```python
from build123d import *

# Parameters (mm, degrees)
SKETCH1_R           = 16
SKETCH1_R_2         = 5
BOSS_EXTRUDE3_DEPTH = 70
CUT_EXTRUDE2_DEPTH  = 16
CUT_EXTRUDE3_DEPTH  = 16
SKETCH7_W           = 34
SKETCH7_H           = 251.612307305
CUT_EXTRUDE4_DEPTH  = 87.5
CUT_EXTRUDE5_DEPTH  = 34
BOSS_EXTRUDE4_START = -38
BOSS_EXTRUDE4_DEPTH = 38
CUT_EXTRUDE6_DEPTH  = 135


with BuildPart() as part:
    # Sketch1 → Boss-Extrude3 (new body)
    with BuildSketch(Plane.XY):
        with BuildLine():
            Line((-18.492879119, 133.036316601), (-18.498498023, 133.025878551))
            ThreePointArc((-18.498498023, 133.025878551), (-22.931133945, 136.748933151), (-27.911859958, 139.698808598))
            Line((-27.911859958, 139.698808598), (-28.859852333, 137.937754807))
            ThreePointArc((-28.859852333, 137.937754807), (-24.623995913, 135.183968868), (-20.885371833, 131.785659496))
            ThreePointArc((-20.885371833, 131.785659496), (-18.192980361, 129.380347747), (-15.794912153, 126.681502565))
            Line((-15.794912153, 126.681502565), (-27.917185271, 110.194914382))
            Line((-27.917185271, 110.194914382), (-24.189891295, 89.250297825))
            ThreePointArc((-24.189891295, 89.250297825), (-23.276240724, 85.794240187), (-23.472804176, 82.224862851))
            ThreePointArc((-23.472804176, 82.224862851), (-68.872718383, -33.767386176), (-52.667247609, -157.269356853))
            ThreePointArc((-52.667247609, -157.269356853), (-50.575514204, -160.492975125), (-47.422535875, -162.689743445))
            ThreePointArc((-47.422535875, -162.689743445), (-9.297986917, -160.884668476), (12.205361962, -129.351423863))
            ThreePointArc((12.205361962, -129.351423863), (11.215393371, -86.524352781), (-3.124290711, -46.157144361))
            ThreePointArc((-3.124290711, -46.157144361), (-18.241573573, 16.806753647), (0.520816468, 78.782211802))
            ThreePointArc((0.520816468, 78.782211802), (0.815698001, 71.975939249), (0.917818465, 65.164047251))
            Line((0.917818465, 65.164047251), (0.943780266, 65.164047251))
            ThreePointArc((0.943780266, 65.164047251), (0.943812795, 65.09180253), (0.943823638, 65.019557802))
            ThreePointArc((0.943823638, 65.019557802), (0.529498651, 60.000787978), (-0.371750777, 55.04624812))
            Line((-0.371750777, 55.04624812), (1.628249223, 55.04624812))
            ThreePointArc((1.628249223, 55.04624812), (2.583543249, 60.061971917), (2.90683401, 65.157612698))
            ThreePointArc((2.90683401, 65.157612698), (2.906823344, 65.229857425), (2.906791346, 65.302102146))
            ThreePointArc((2.906791346, 65.302102146), (2.809025603, 72.019742255), (2.526858646, 78.732165705))
            ThreePointArc((2.526858646, 78.732165705), (-2.46660039, 104.447349639), (-14.187653785, 127.874304738))
            ThreePointArc((-14.187653785, 127.874304738), (-16.217340169, 130.557833748), (-18.492879119, 133.036316601))
        make_face()
        with Locations((-30.170544826, -123.552650361)):
            Circle(SKETCH1_R, mode=Mode.SUBTRACT)
        with Locations((-30.170544826, -85.552650361)):
            Circle(SKETCH1_R_2, mode=Mode.SUBTRACT)
    extrude(amount=BOSS_EXTRUDE3_DEPTH)

    # Sketch4 → Cut-Extrude2 (cut)
    with BuildSketch(Plane(origin=(0, 0, 0), x_dir=(-1, 0, 0), z_dir=(0, 0, -1))):
        with BuildLine():
            Line((27.917185271, 110.194914382), (15.794912153, 126.681502565))
            ThreePointArc((15.794912153, 126.681502565), (4.373722035, 103.843429765), (-0.520816468, 78.782211802))
            ThreePointArc((-0.520816468, 78.782211802), (18.241573573, 16.806753647), (3.124290711, -46.157144361))
            ThreePointArc((3.124290711, -46.157144361), (-11.215393371, -86.524352781), (-12.205361962, -129.351423863))
            ThreePointArc((-12.205361962, -129.351423863), (9.297986917, -160.884668476), (47.422535875, -162.689743445))
            ThreePointArc((47.422535875, -162.689743445), (50.575514204, -160.492975125), (52.667247609, -157.269356853))
            ThreePointArc((52.667247609, -157.269356853), (68.872718383, -33.767386176), (23.472804176, 82.224862851))
            ThreePointArc((23.472804176, 82.224862851), (23.276240724, 85.794240187), (24.189891295, 89.250297825))
            Line((24.189891295, 89.250297825), (27.917185271, 110.194914382))
        make_face()
    extrude(amount=-CUT_EXTRUDE2_DEPTH, mode=Mode.SUBTRACT)

    # Sketch5 → Cut-Extrude3 (cut)
    with BuildSketch(Plane.XY.offset(70)):
        with BuildLine():
            Line((-15.794912153, 126.681502565), (-106.344691982, 77.715450511))
            Line((-106.344691982, 77.715450511), (-99.056785555, -184.356883009))
            Line((-99.056785555, -184.356883009), (38.776437557, -199.728468659))
            Line((38.776437557, -199.728468659), (9.520070812, 37.732141377))
            Line((9.520070812, 37.732141377), (-2.731904314, 53.720528852))
            Line((-2.731904314, 53.720528852), (0.520816468, 78.782211802))
            ThreePointArc((0.520816468, 78.782211802), (-4.80960476, 103.694956914), (-15.794912153, 126.681502565))
        make_face()
    extrude(amount=-CUT_EXTRUDE3_DEPTH, mode=Mode.SUBTRACT)

    # Sketch7 → Cut-Extrude4 (cut, symmetric)
    with BuildSketch(Plane(origin=(0, 0, 0), x_dir=(0, 0, -1), z_dir=(1, 0, 0))):
        with Locations((-35, -70.759905532)):
            Rectangle(SKETCH7_W, SKETCH7_H)
    extrude(amount=CUT_EXTRUDE4_DEPTH, both=True, mode=Mode.SUBTRACT)

    # Sketch8 → Cut-Extrude5 (cut)
    with BuildSketch(Plane(origin=(0, 0, 52), x_dir=(-1, 0, 0), z_dir=(0, 0, -1))):
        with BuildLine():
            Line((15.794912153, 126.681502565), (103.727403684, 77.715450511))
            Line((103.727403684, 77.715450511), (65.201238751, -183.077529844))
            Line((65.201238751, -183.077529844), (-41.355481636, -162.759511126))
            Line((-41.355481636, -162.759511126), (-12.07256107, 35.463700067))
            Line((-12.07256107, 35.463700067), (7.253704803, 49.814895562))
            Line((7.253704803, 49.814895562), (-0.520816468, 78.782211802))
            ThreePointArc((-0.520816468, 78.782211802), (4.735822291, 103.720089118), (15.794912153, 126.681502565))
        make_face()
    extrude(amount=CUT_EXTRUDE5_DEPTH, mode=Mode.SUBTRACT)

    # Sketch9 → Boss-Extrude4 (add)
    with BuildSketch(Plane.XY.offset(54).offset(BOSS_EXTRUDE4_START)):
        with BuildLine():
            Line((-8.381762523, 61.719660218), (-9.752633242, 63.175927181))
            ThreePointArc((-9.752633242, 63.175927181), (-17.943118256, 36.524072516), (-20.049083933, 8.721728902))
            Line((-20.049083933, 8.721728902), (-18.21549071, 8.787163684))
            ThreePointArc((-18.21549071, 8.787163684), (-16.213088176, 35.794856709), (-8.381762523, 61.719660218))
        make_face()
    extrude(amount=BOSS_EXTRUDE4_DEPTH)

    # Sketch11 → Cut-Extrude6 (cut)
    with BuildSketch(Plane.XY.offset(54)):
        with BuildLine():
            Line((-50.185023147, -28.598308606), (-19.867347918, -59.472801703))
            ThreePointArc((-19.867347918, -59.472801703), (-19.113609075, -62.364150109), (-21.230995297, -64.472394267))
            Line((-21.230995297, -64.472394267), (-53.847995089, -73.217282749))
            ThreePointArc((-53.847995089, -73.217282749), (-56.418775041, -72.724188951), (-57.623794539, -70.400403449))
            ThreePointArc((-57.623794539, -70.400403449), (-57.31161949, -50.287283004), (-55.294991455, -30.273081081))
            ThreePointArc((-55.294991455, -30.273081081), (-53.259893991, -27.84944683), (-50.185023147, -28.598308606))
        make_face()
        with BuildLine():
            Line((-22.762737067, -45.106159898), (-51.405782898, -15.937052632))
            ThreePointArc((-51.405782898, -15.937052632), (-52.148347837, -14.664421133), (-52.195447125, -13.191744903))
            ThreePointArc((-52.195447125, -13.191744903), (-47.4284487, 5.029431131), (-41.229607384, 22.814534346))
            ThreePointArc((-41.229607384, 22.814534346), (-40.234764305, 24.117966642), (-38.703222855, 24.703653665))
            Line((-38.703222855, 24.703653665), (-32.552921731, 25.249075291))
            ThreePointArc((-32.552921731, 25.249075291), (-30.190849915, 24.406103869), (-29.294390199, 22.063809255))
            ThreePointArc((-29.294390199, 22.063809255), (-27.47951255, -10.554827918), (-17.882279592, -41.782418145))
            ThreePointArc((-17.882279592, -41.782418145), (-18.933525001, -45.483819939), (-22.762737067, -45.106159898))
        make_face()
    extrude(amount=-CUT_EXTRUDE6_DEPTH, mode=Mode.SUBTRACT)


solid = part.part
```
Input: part model. Units: mm. Frame: model coordinates. A direction names the side the tool comes from. Coordinates: 2 decimals unless noted, no trailing zeros. Loops run counter-clockwise (first coordinate to the right, second up) from the corner with the lowest first, then second, coordinate; pieces in that order, holes last. Notation, with made-up numbers: (72, 35) -> (108, 35) arc R33 ccw to (108, 68) -> close; hole circle Ø11 at (36.25, -18). An arc over 180 degrees is marked (long way). Use a Markdown table: item, result.
1) Access query for faces 1 (the flat face through (-21.771, 118.554, 16.986)), 2 (the flat face through (-36.88, -30.73, 17.01)), 3 (the cylindrical face through (-9.78, -161.15, 16.99)). Directions: +Z, -Z, +X, -X, +Y, -Y. A direction counts if a zero-diameter tool reaches every point of the face in a straight line with its end or side. Return the directions, or none.
Results found:
| item | result |
|---|---|
| face 1 | +Z, -Z, -X |
| face 2 | +Z, -Z |
| face 3 | +Z, -Z, -Y |
2) Cut plane D-D (y = -96). Return the cut outline in (x, z), then the cut area to 3 significant figures.
Results found:
| item | result |
|---|---|
| outline | (-68.66, 16) -> (12.62, 16) -> (12.62, 18) -> (-68.66, 18) -> close; (-68.66, 52) -> (12.62, 52) -> (12.62, 54) -> (-68.66, 54) -> close |
| area | 325 mm2 |
3) Contact query for flat-ended pins moving along their axis: pin 1 (8 mm diameter, centred on x = -27, y = 69.5, fed in from +Z); pin 2 (12 mm diameter, centred on x = -48.5, y = -21, fed in from -Z); pin 3 (1 mm diameter, centred on x = -4.5, z = 17, fed in from +Y). Output: stop coordinate, or through.
Results found:
| item | result |
|---|---|
| pin 1 | stops at z = 54 |
| pin 2 | stops at z = 16 |
| pin 3 | stops at y = 111.08 |
4) Pull-direction query (Z, two-part tool) for faces 4 (the flat face through (-20, -50, 16)), 5 (the cylindrical face through (2.575, 59.991, 34.51)), 6 (the cylindrical face through (-17.87, 36.91, 34.76)); classes: released by +Z, released by -Z, zero draft, split by the parting line, or undercut.
Results found:
| item | result |
|---|---|
| face 4 | released by -Z |
| face 5 | zero draft |
| face 6 | undercut |
5) Material intervals for line 1 along Z through (x, y) = (-63.5, -79); line 2 along X through (y, z) = (90.5, 58.5); line 3 along Y through (x, z) = (-11, 57.5), sorted ascending. Write a range as from..to.
Results found:
| item | result |
|---|---|
| line 1 | z = 16..18, 52..54 |
| line 2 | x = -1.22..1.14 |
| line 3 | y = 118.28..122.89 |
6) Cut plane B-B (x = -61). Return the cut outline in (y, z), then the cut area to 3 significant figures.
Results found:
| item | result |
|---|---|
| outline | (-133.02, 16) -> (4.98, 16) -> (4.98, 18) -> (-133.02, 18) -> close; (-133.02, 52) -> (4.98, 52) -> (4.98, 54) -> (-133.02, 54) -> close |
| area | 552 mm2 |
